The model under review builds one solid part; all positions refer to its coordinate system, in mm. Face numbers are marked on the shaded views. A direction names the side the tool comes from. Round coordinates to 2 decimals unless told otherwise and drop trailing zeros. Order: outer loops, then holes, each group sorted by start corner. A loop starts at its lowest first (then second) coordinate and runs counter-clockwise, first axis right, second up.
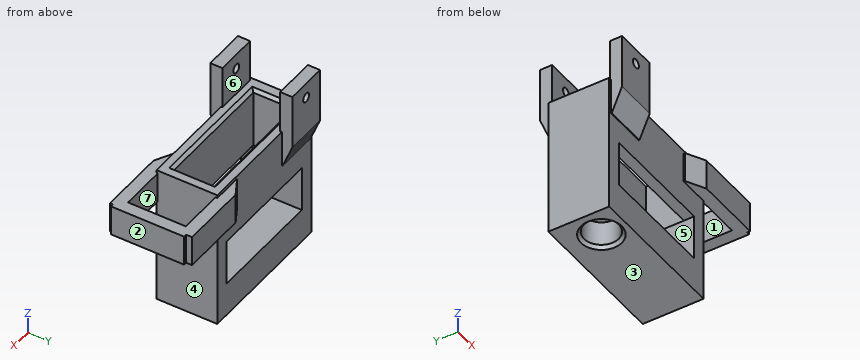
from build123d import *

# Parameters (mm, degrees)
BOX_W             = 23.85
BOX_H             = 10
BOX_DEPTH         = 23
BOX001_W          = 20
BOX001_H          = 6.55
BOX001_DEPTH      = 9.9
BOX002_W          = 19
BOX002_H          = 15
BOX002_DEPTH      = 7.5
CHAMFER_SIZE      = 0.5
CYLINDER_R        = 2.85
CYLINDER_DEPTH    = 4.5
CHAMFER001_SIZE   = 0.5
BOX003_W          = 7
BOX003_H          = 2
BOX003_DEPTH      = 13
CHAMFER002_SIZE2  = 4
CHAMFER002_SIZE   = 1.7
BOX004_W          = 7
BOX004_H          = 2
BOX004_DEPTH      = 13
CYLINDER001_R     = 0.75
CYLINDER001_DEPTH = 15
CHAMFER003_SIZE2  = 4
CHAMFER003_SIZE   = 1.6
BOX005_W          = 5
BOX005_H          = 2
BOX005_DEPTH      = 14
CHAMFER004_SIZE2  = 3
CHAMFER004_SIZE   = 1.6
BOX006_W          = 5
BOX006_H          = 2
BOX006_DEPTH      = 14
CHAMFER005_SIZE2  = 3
CHAMFER005_SIZE   = 1.69
BOX007_W          = 5
BOX007_H          = 12
BOX007_DEPTH      = 2


with BuildPart() as part:
    # Box → Box (join)
    with BuildSketch(Plane.XY):
        with Locations((11.925, 5)):
            Rectangle(BOX_W, BOX_H)
    extrude(amount=BOX_DEPTH)

    # Box001 → Box001 (cut)
    with BuildSketch(Plane(origin=(2, 1.7, 13.1), x_dir=(1, 0, 0), z_dir=(0, 0, 1))):
        with Locations((10, 3.275)):
            Rectangle(BOX001_W, BOX001_H)
    extrude(amount=BOX001_DEPTH, mode=Mode.SUBTRACT)

    # Box002 → Box002 (cut)
    with BuildSketch(Plane(origin=(2.5, -2.8, 5.6), x_dir=(1, 0, 0), z_dir=(0, 0, 1))):
        with Locations((9.5, 7.5)):
            Rectangle(BOX002_W, BOX002_H)
    extrude(amount=BOX002_DEPTH, mode=Mode.SUBTRACT)

    # Chamfer
    chamfer_edges = [part.edges().sort_by_distance(p)[0] for p in [
        (12, 8.25, 23),
        (22, 4.975, 23),
        (12, 1.7, 23),
        (2, 4.975, 23),
    ]]
    chamfer(chamfer_edges, length=CHAMFER_SIZE)

    # Cylinder → Cylinder (cut)
    with BuildSketch(Plane(origin=(4.5, 4.2, 4.5), x_dir=(1, 0, 0), z_dir=(0, 0, -1))):
        Circle(CYLINDER_R)
    extrude(amount=CYLINDER_DEPTH, mode=Mode.SUBTRACT)

    # Chamfer001
    chamfer001_edges = [part.edges().sort_by_distance(p)[0] for p in [
        (1.65, 4.2, 0),
    ]]
    chamfer(chamfer001_edges, length=CHAMFER001_SIZE)

    # Box003 → Box003 (join)
    with BuildSketch(Plane(origin=(0.5, -1.8, 17), x_dir=(1, 0, 0), z_dir=(0, 0, 1))):
        with Locations((3.5, 1)):
            Rectangle(BOX003_W, BOX003_H)
    extrude(amount=BOX003_DEPTH)

    # Chamfer002
    chamfer002_edges = [part.edges().sort_by_distance(p)[0] for p in [
        (4, -1.8, 17),
    ]]
    chamfer002_side = part.faces().sort_by_distance((4, -0.9, 17))[0]
    chamfer(chamfer002_edges, length=CHAMFER002_SIZE, length2=CHAMFER002_SIZE2, reference=chamfer002_side)

    # Box004 → Box004 (join)
    with BuildSketch(Plane(origin=(0.5, 9.7, 17), x_dir=(1, 0, 0), z_dir=(0, 0, 1))):
        with Locations((3.5, 1)):
            Rectangle(BOX004_W, BOX004_H)
    extrude(amount=BOX004_DEPTH)

    # Cylinder001 → Cylinder001 (cut)
    with BuildSketch(Plane(origin=(4, -2.8, 27.5), x_dir=(-1, 0, 0), z_dir=(0, 1, 0))):
        Circle(CYLINDER001_R)
    extrude(amount=CYLINDER001_DEPTH, mode=Mode.SUBTRACT)

    # Chamfer003
    chamfer003_edges = [part.edges().sort_by_distance(p)[0] for p in [
        (4, 11.7, 17),
    ]]
    chamfer003_side = part.faces().sort_by_distance((4, 10.85, 17))[0]
    chamfer(chamfer003_edges, length=CHAMFER003_SIZE, length2=CHAMFER003_SIZE2, reference=chamfer003_side)

    # Box005 → Box005 (join)
    with BuildSketch(Plane(origin=(18.85, -1.8, 22.5), x_dir=(0, 0, -1), z_dir=(1, 0, 0))):
        with Locations((2.5, 1)):
            Rectangle(BOX005_W, BOX005_H)
    extrude(amount=BOX005_DEPTH)

    # Chamfer004
    chamfer004_edges = [part.edges().sort_by_distance(p)[0] for p in [
        (18.85, -1.8, 20),
    ]]
    chamfer004_side = part.faces().sort_by_distance((18.85, -0.9, 20))[0]
    chamfer(chamfer004_edges, length=CHAMFER004_SIZE, length2=CHAMFER004_SIZE2, reference=chamfer004_side)

    # Box006 → Box006 (join)
    with BuildSketch(Plane(origin=(18.85, 9.7, 22.5), x_dir=(0, 0, -1), z_dir=(1, 0, 0))):
        with Locations((2.5, 1)):
            Rectangle(BOX006_W, BOX006_H)
    extrude(amount=BOX006_DEPTH)

    # Chamfer005
    chamfer005_edges = [part.edges().sort_by_distance(p)[0] for p in [
        (18.85, 11.7, 20),
    ]]
    chamfer005_side = part.faces().sort_by_distance((18.85, 10.85, 20))[0]
    chamfer(chamfer005_edges, length=CHAMFER005_SIZE, length2=CHAMFER005_SIZE2, reference=chamfer005_side)

    # Box007 → Box007 (join)
    with BuildSketch(Plane(origin=(31.35, -1.3, 22.5), x_dir=(0, 0, -1), z_dir=(1, 0, 0))):
        with Locations((2.5, 6)):
            Rectangle(BOX007_W, BOX007_H)
    extrude(amount=BOX007_DEPTH)


solid = part.part
(1) We need section D-D (z = 27.5). Give the boundary of the cut face in (x, y).
(2) The part is to be moulded in two halves that separate along X. For the marked faces 1, 2, 3 and 4, say which applies: pulls with the +X half, pulls with the -X half, needs draft (parallel to the pull), parting line crosses it, or undercut.
(3) To check wall thickness, follow L1, parallel to X at y = 5.5, z = 21.5; L2, parallel to X at y = 10.9, z = 27.5; L3, parallel to Y at x = 6.5, z = 15.5. State the ranges of each line that lie inside material, in increasing order.
(4) We need section B-B (x = 18). Give the boundary of the cut face in (y, z).
(5) Tool access review of the marked faces 5, 6 and 7: name each direction out of +Z, -Z, +X, -X, +Y, -Y from which nothing blocks a thin tool from reaching the whole face with its end or side.
(6) We need section C-C (x = 29). Give the boundary of the cut face in (y, z).
(7) We need section A-A (z = 7.75). Give the boundary of the cut face in (x, y).
(8) Clearance check with flat-ended pins moving along their axes: P1, Ø3, axis at x = 13.5, z = 12, coming from the -Y side; P2, Ø3.5, axis at x = 4.5, y = 4.2, coming from the -Z side; P3, Ø6, axis at x = 16, y = 7.5, coming from the -Z side; P4, Ø5, axis at x = 17.5, y = 3, coming from the +Z side. State where each tip first meets the part, or that it passes through.
Verdict:
1. outline: (0.5, -1.8) - (3.25, -1.8) - (3.25, 0.2) - (0.5, 0.2) - close; (0.5, 9.7) - (3.25, 9.7) - (3.25, 11.7) - (0.5, 11.7) - close; (4.75, -1.8) - (7.5, -1.8) - (7.5, 0.2) - (4.75, 0.2) - close; (4.75, 9.7) - (7.5, 9.7) - (7.5, 11.7) - (4.75, 11.7) - close
2. face 1: undercut
2. face 2: pulls with the +X half
2. face 3: needs draft
2. face 4: undercut
3. L1: x = 0 to 2, 22 to 23.85, 31.35 to 33.35
3. L2: x = 0.5 to 3.25, 4.75 to 7.5
3. L3: y = 0 to 1.7, 8.25 to 10
4. outline: (0, 0) - (10, 0) - (10, 5.6) - (0, 5.6) - close; (0, 13.1) - (1.7, 13.1) - (1.7, 22.5) - (1.2, 23) - (0, 23) - close; (8.25, 13.1) - (10, 13.1) - (10, 23) - (8.75, 23) - (8.25, 22.5) - close
5. face 5: +Y, -Y
5. face 6: +Z, +X, -X
5. face 7: +Z, -Z
6. outline: (-1.8, 17.5) - (0.2, 17.5) - (0.2, 22.5) - (-1.8, 22.5) - close; (9.7, 17.5) - (11.7, 17.5) - (11.7, 22.5) - (9.7, 22.5) - close
7. outline: (0, 0) - (2.5, 0) - (2.5, 10) - (0, 10) - close; (21.5, 0) - (23.85, 0) - (23.85, 10) - (21.5, 10) - close
8. P1: stops at y = 0
8. P2: stops at z = 4.5
8. P3: stops at z = 0
8. P4: stops at z = 23
